Source: CAD feature listing. Evaluate the final solid. Frame: model axes, mm. Face numbers are marked on the shaded views. A direction names the side the tool comes from. Round coordinates to 2 decimals unless told otherwise and drop trailing zeros. Order: outer loops, then holes, each group sorted by start corner. A loop starts at its lowest first (then second) coordinate and runs counter-clockwise, first axis right, second up. Notation, with made-up numbers: M 30,-15 L 84,-15 A16 ccw 84,11 Z; hole C 5.5,64.5 d2. An arc over 180 degrees is marked long. Answer in a Markdown table with one row per item. Add a question column.
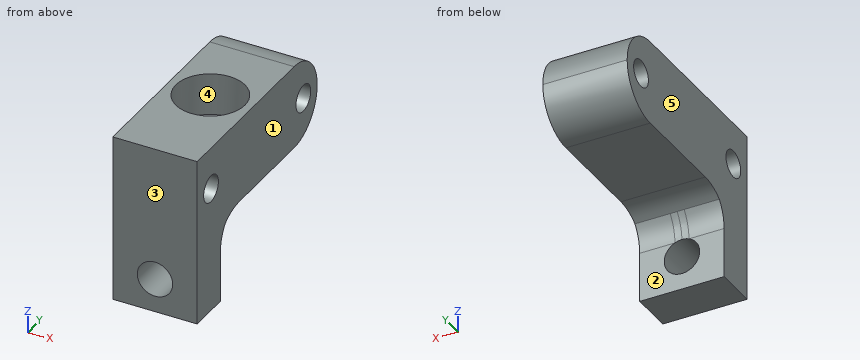
```python
from build123d import *

# Parameters (mm, degrees)
ESQUISSE1_W             = 10
ESQUISSE1_H             = 26
ESQUISSE1_R             = 4.1
BOSS_EXTRU_1_DEPTH      = 10
ESQUISSE2_R             = 1.6
ENL_V_MAT_EXTRU_1_DEPTH = 10
ESQUISSE3_W             = 10
ESQUISSE3_H             = 10
BOSS_EXTRU_2_DEPTH      = 5
CHANFREIN1_SIZE         = 2
ESQUISSE4_R             = 2.1
ENL_V_MAT_EXTRU_2_DEPTH = 5
ESQUISSE5_R             = 4.106671815
BOSS_EXTRU_3_DEPTH      = 5
CONG_1_R                = 5


# Some blends are built 0.0001 mm under size
with BuildPart() as part:
    # Esquisse1 → Boss.-Extru.1 (new body)
    with BuildSketch(Plane.XY):
        with Locations((5, 13)):
            Rectangle(ESQUISSE1_W, ESQUISSE1_H)
        with Locations((5, 12)):
            Circle(ESQUISSE1_R, mode=Mode.SUBTRACT)
    extrude(amount=BOSS_EXTRU_1_DEPTH)

    # Esquisse2 → Enlèv. mat.-Extru.1 (cut)
    with BuildSketch(Plane.ZY):
        with Locations((5, 23)):
            Circle(ESQUISSE2_R)
        with Locations((5, 3)):
            Circle(ESQUISSE2_R)
    extrude(amount=-ENL_V_MAT_EXTRU_1_DEPTH, mode=Mode.SUBTRACT)

    # Esquisse3 → Boss.-Extru.2 (add)
    with BuildSketch(Plane.XZ):
        with Locations((5, -5)):
            Rectangle(ESQUISSE3_W, ESQUISSE3_H)
    extrude(amount=-BOSS_EXTRU_2_DEPTH)

    # Chanfrein1
    chanfrein1_edges = [part.edges().sort_by_distance(p)[0] for p in [
        (5, 5, 0),
    ]]
    chamfer(chanfrein1_edges, length=CHANFREIN1_SIZE)

    # Esquisse4 → Enlèv. mat.-Extru.2 (cut)
    with BuildSketch(Plane(origin=(0, 5, 0), x_dir=(1, 0, 0), z_dir=(0, 1, 0))):
        with Locations(Location((5, 6, 0), (0, 0, 270))):
            Circle(ESQUISSE4_R)
    extrude(amount=-ENL_V_MAT_EXTRU_2_DEPTH, mode=Mode.SUBTRACT)

    # Esquisse5 → Boss.-Extru.3 (add)
    with BuildSketch(Plane(origin=(0, 0, 0), x_dir=(-1, 0, 0), z_dir=(0, 0, -1))):
        with Locations((-5, 12)):
            Circle(ESQUISSE5_R)
    extrude(amount=-BOSS_EXTRU_3_DEPTH)

    # Congé1
    cong_1_edges = [part.edges().sort_by_distance(p)[0] for p in [
        (5, 5, -2),
    ]]
    fillet(cong_1_edges, radius=CONG_1_R)
    cong_1_2_edges = [part.edges().sort_by_distance(p)[0] for p in [
        (5, 26, 0),
    ]]
    fillet(cong_1_2_edges, radius=CONG_1_R)
    cong_1_3_edges = [part.edges().sort_by_distance(p)[0] for p in [
        (5, 26, 10),
    ]]
    fillet(cong_1_3_edges, radius=CONG_1_R - 0.0001)  # a hair under: the kernel refuses the full size
    # the kernel refuses this fillet: 5 mm, written as the material it adds along each edge
    with BuildSketch(Plane(origin=(10, 7, 0), x_dir=(0, 1, 0), z_dir=(-1, 0, 0))) as cong_1_4_piece_1:
        with BuildLine():
            CenterArc((CONG_1_R * 0.414213562373, CONG_1_R), CONG_1_R, 225, 45)
            Line((-CONG_1_R * 0.292893218813, CONG_1_R * 0.292893218813), (-CONG_1_R * 0.307035354437, CONG_1_R * 0.27875108319))
            Line((-CONG_1_R * 0.307035354437, CONG_1_R * 0.27875108319), (-CONG_1_R * 0.00828427124746, -CONG_1_R * 0.02))
            Line((-CONG_1_R * 0.00828427124746, -CONG_1_R * 0.02), (CONG_1_R * 0.414213562373, -CONG_1_R * 0.02))
            Line((CONG_1_R * 0.414213562373, -CONG_1_R * 0.02), (CONG_1_R * 0.414213562373, 0))
        make_face()
    extrude(amount=10)


solid = part.part
```
(1) Cut plane B-B (z = -6). Return loops of the section in (x, y).
(2) Cut plane D-D (z = 5.5). Return loops of the section in (x, y), and give its area (3 significant figures).
(3) Pin query (flat end, axial travel): pin 1 (2 mm diameter, centred on x = 9, y = 21, fed in from -Z); pin 2 (2 mm diameter, centred on x = 2.5, z = -6, fed in from +Y). Return the tip coordinate at first contact, or that it passes through.
(4) Cut plane A-A (y = 3). Return loops of the section in (x, z).
(5) Cut plane C-C (y = 12). Return loops of the section in (x, z).
(6) Access query for the marked faces 1 and 2. Directions: +Z, -Z, +X, -X, +Y, -Y. A direction counts if a zero-diameter tool reaches every point of the face in a straight line with its end or side. Return the directions, or none.
(7) Line query: line 1 (Z direction, x = 3.75, y = 19.5); line 2 (Y direction, x = 6.75, z = 8.5); line 3 (Y direction, x = 7.5, z = -4.5). Output: solid intervals per line, ascending. Write a range as from..to.
(8) Draft query along X for the marked faces 3, 4 and 5. Return one class per face: +X half, -X half, draft (parallel to the pull), parting line (faces both ways), or undercut.
Answer list:
| question | item | result |
|---|---|---|
| 1 | outline | M 0,0 L 2.9,0 L 2.9,5 L 0,5 Z; M 7.1,0 L 10,0 L 10,5 L 7.1,5 Z |
| 2 | outline | M 0,0 L 10,0 L 10,1.48 L 0,1.48 Z; M 0,4.52 L 10,4.52 L 10,21.48 L 0,21.48 Z; M 0,24.52 L 10,24.52 L 10,25.97 L 0,25.97 Z; hole C 5,12 d8.2 |
| 2 | area | 146 mm² |
| 3 | pin 1 | z = 0 |
| 3 | pin 2 | y = 5 |
| 4 | outline | M 0,-10 L 10,-10 L 10,3.4 L 0,3.4 Z; M 0,6.6 L 10,6.6 L 10,10 L 0,10 Z; hole C 5,-6 d4.2 |
| 5 | outline | M 0,0 L 10,0 L 10,10 L 9.1,10 L 9.1,5 L 0.9,5 L 0.9,10 L 0,10 Z |
| 6 | face 1 | +Z, -Z, +X, +Y, -Y |
| 6 | face 2 | -Z, +X, -X, +Y |
| 7 | line 1 | 0..10 |
| 7 | line 2 | 0..8.29, 15.71..24.57 |
| 7 | line 3 | 0..5 |
| 8 | face 3 | draft |
| 8 | face 4 | undercut |
| 8 | face 5 | -X half |
